Could you check a few things on this model? Use its own coordinates, in mm. A direction names the side the tool comes from. Give positions to 0.01 mm unless a question says otherwise; leave off trailing zeros. Loops run counter-clockwise (first coordinate to the right, second up) from the corner with the lowest first, then second, coordinate; pieces in that order, holes last.
1. Imagine slicing it at B-B (z = -58). List the corners of the cut face in (x, y) for me, plus the area to 3 significant figures.
2. I need wall thicknesses on line 1 along Z through (x, y) = (-6.5, 9.5); line 2 along Z through (x, y) = (-12, 7); line 3 along Y through (x, z) = (1.5, -52). Which ranges of each line are inside material? Lowest first, please.
3. For P1, Ø1, axis at x = -5, z = -15, coming from the +Y side; P2, Ø1.5, axis at x = -7.5, y = -11, coming from the -Z side; P3, Ø1, axis at y = -11, z = -34.5, coming from the -X side; P4, Ø8.5, axis at x = 6.5, y = -0.5, coming from the +Z side, each with a flat end and sliding along its axis, tell me the tip position at first contact or that it passes through.
4. For faces 1 (the flat face through (5, 10, -56)), 2 (the cylindrical face through (5.19, 9.98, -16.52)), 3 (the cylindrical face through (6.58, 12.64, -2.54)), which set-ups out of +Z, -Z, +X, -X, +Y, -Y let a thin tool reach every point of the face, with its end or its side?
5. Thinking about a two-plate mould opening in Z: for faces 4 (the flat face through (0, 0, -63)), 5 (the cylindrical face through (-2.93, 13.18, -51.94)), 6 (the cylindrical face through (6.691, 12.864, -43.542)), which applies, +Z half, -Z half, draft (parallel to the pull), parting line (faces both ways), or undercut?
6. Imagine slicing it at A-A (z = -39). List the corners of the cut face in (x, y) for me, plus the area to 3 significant figures.
```python
from build123d import *

# Parameters (mm, degrees)
SKETCH1_W     = 5
SKETCH1_H     = 14.25
SKETCH1_W_2   = 3
SKETCH1_H_2   = 11.25
SKETCH1_W_3   = 6
SKETCH1_H_3   = 14.5
SKETCH1_W_4   = 7
SKETCH1_H_4   = 11
CHAMFER1_SIZE = 1
CHAMFER2_SIZE = 0.5


with BuildPart() as part:
    # Sketch1 → Revolve1 (revolve)
    with BuildSketch(Plane(origin=(0, 0, 0), x_dir=(0, 0, -1), z_dir=(1, 0, 0)), mode=Mode.PRIVATE) as revolve1_sk:
        with Locations((2.5, 7.125)):
            Rectangle(SKETCH1_W, SKETCH1_H)
        Polygon((5, 13.25), (5, 0), (13.5, 0), (13.5, 11.25), (13.5, 13.25), align=None)
        Polygon((13.5, 11.25), (13.5, 0), (15, 0), (15, 11.25), (15, 14.25), (13.5, 14.25), (13.5, 13.25), align=None)
        with Locations((16.5, 5.625)):
            Rectangle(SKETCH1_W_2, SKETCH1_H_2)
        Polygon((18, 11.25), (18, 0), (38, 0), (38, 14.25), (18, 14.25), align=None)
        Polygon((38, 14.25), (38, 0), (40.5, 0), (40.5, 14.5), (40.5, 15.25), (38, 15.25), align=None)
        with Locations((43.5, 7.25)):
            Rectangle(SKETCH1_W_3, SKETCH1_H_3)
        Polygon((46.5, 14.5), (46.5, 0), (48, 0), (48, 13.5), (48, 15.25), (46.5, 15.25), align=None)
        Polygon((48, 13.5), (48, 0), (56, 0), (56, 11), (56, 13.5), align=None)
        with Locations((59.5, 5.5)):
            Rectangle(SKETCH1_W_4, SKETCH1_H_4)
    revolve(revolve1_sk.sketch.rotate(Axis((0, 0, -5), (0, 0, -1)), 90), axis=Axis((0, 0, -5), (0, 0, -1)))

    # Chamfer1
    chamfer1_edges = [part.edges().sort_by_distance(p)[0] for p in [
        (-14.25, 0, -18),
    ]]
    chamfer(chamfer1_edges, length=CHAMFER1_SIZE)

    # Chamfer2
    chamfer2_edges = [part.edges().sort_by_distance(p)[0] for p in [
        (-14.25, 0, -15),
    ]]
    chamfer(chamfer2_edges, length=CHAMFER2_SIZE)


solid = part.part
```
Derived:
1. outline: circle Ø22 at (0, 0)
1. area: 380 mm2
2. line 1: z = -56 to -18, -15 to 0
2. line 2: z = -48 to -18.64, -14.86 to -13.5, -5 to 0
2. line 3: y = -13.42 to 13.42
3. P1: stops at y = 13.37
3. P2: stops at z = -56
3. P3: stops at x = -9.63
3. P4: stops at z = 0
4. face 1: -Z
4. face 2: none
4. face 3: +Z
5. face 4: -Z half
5. face 5: draft
5. face 6: undercut
6. outline: circle Ø30.5 at (0, 0)
6. area: 731 mm2
